Job drawing, mm, ordinate dimensions from the low corner. One solid piece. A direction names the side the tool comes from. Coordinates: 2 decimals unless noted, no trailing zeros. Order: outer loops, then holes, each group sorted by start corner. A loop starts at its lowest first (then second) coordinate and runs counter-clockwise, first axis right, second up. Notation, with made-up numbers: (45.25, 44) - (95.25, 44) arc R27 cw to (95.25, 77) - close; hole circle Ø11 at (-10.75, 73.5). An arc over 180 degrees is marked (long way). Return JSON: item names as keys, results as strings.
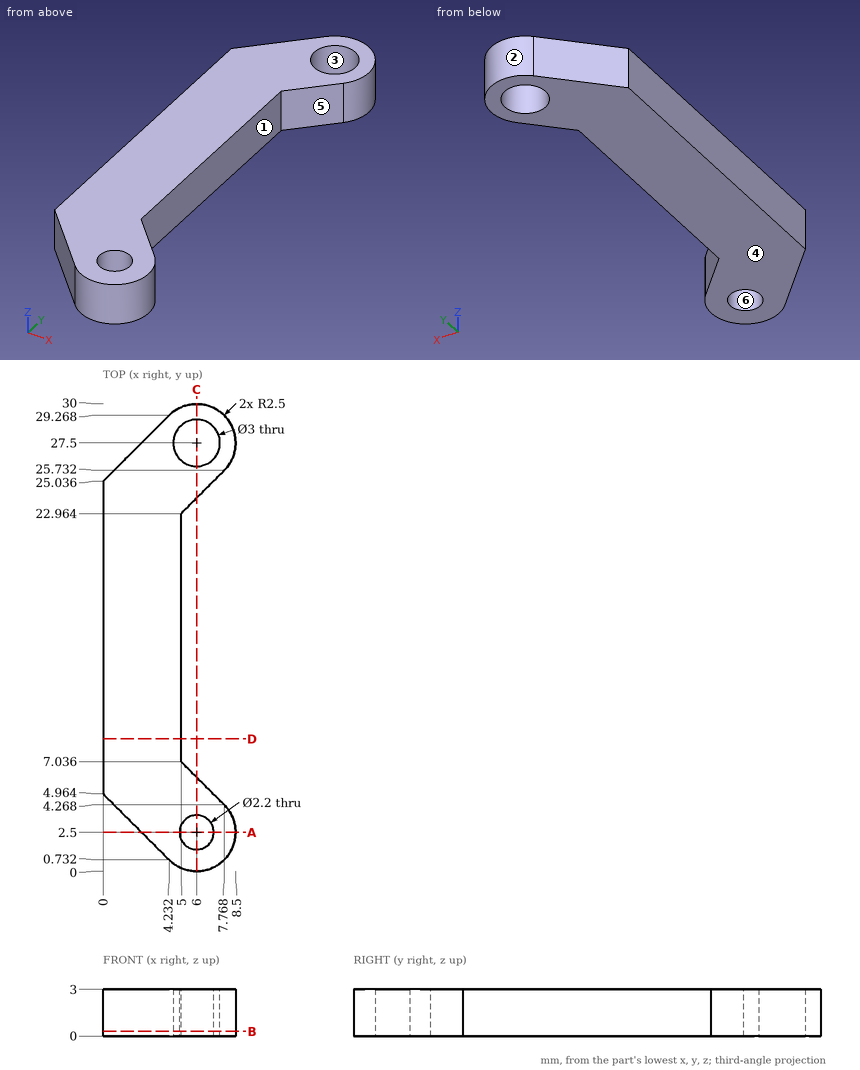
1. Cut at D-D on y = 8.5. Give the cut face in (x, z), plus the area to 3 significant figures.
Check values:
{"outline": "(0, 0) - (5, 0) - (5, 3) - (0, 3) - close", "area": "15.0 mm²"}
2. Mould opens along X. For the marked faces 3, 4, 5 and 6 say: pulls with the +X half, pulls with the -X half, needs draft (parallel to the pull), parting line crosses it, or undercut.
Check values:
{"face 3": "undercut", "face 4": "needs draft", "face 5": "pulls with the +X half", "face 6": "undercut"}
3. Cut at C-C on x = 6. Give the cut face in (y, z) (1 decimal).
Check values:
{"outline": "(0, 0) - (1.4, 0) - (1.4, 3) - (0, 3) - close; (3.6, 0) - (6, 0) - (6, 3) - (3.6, 3) - close; (24, 0) - (26, 0) - (26, 3) - (24, 3) - close; (29, 0) - (30, 0) - (30, 3) - (29, 3) - close"}
4. Drop flat-ended pins along their axis: pin 1 (3.5 mm diameter, centred on x = 6, y = 2.5, fed in from +Z); pin 2 (1 mm diameter, centred on y = 22.5, z = 2.5, fed in from +X) (1 decimal); pin 3 (1.5 mm diameter, centred on y = 24, z = 2, fed in from +X) (1 decimal). Give the stop position or say it passes through.
Check values:
{"pin 1": "z = 3", "pin 2": "x = 5", "pin 3": "x = 6.8"}
5. Cut at B-B on z = 0.3. Give the cut face in (x, y) (1 decimal), plus the area to 3 significant figures.
Check values:
{"outline": "(0, 5) - (4.2, 0.7) arc R2.5 ccw to (7.8, 4.3) - (5, 7) - (5, 23) - (7.8, 25.7) arc R2.5 ccw to (4.2, 29.3) - (0, 25) - close; hole circle Ø3 at (6, 27.5); hole circle Ø2.2 at (6, 2.5)", "area": "148 mm²"}
6. Tool access for the marked faces 1 and 2: list every direction of +Z, -Z, +X, -X, +Y, -Y with a clear straight run to the whole face (end or side of a thin tool).
Check values:
{"face 1": "+Z, -Z, +X", "face 2": "+Z, -Z"}
7. Probe L1, parallel to Y at x = 6, z = 2.1 (1 decimal); L2, parallel to X at y = 25, z = 2.55 (1 decimal); L3, parallel to X at y = 8.5, z = 1.85. List the from-to ranges inside material, lowest first.
Check values:
{"L1": "0 to 1.4, 3.6 to 6, 24 to 26, 29 to 30", "L2": "0 to 7", "L3": "0 to 5"}
8. Cut at A-A on y = 2.5. Give the cut face in (x, z) (1 decimal).
Check values:
{"outline": "(2.5, 0) - (4.9, 0) - (4.9, 3) - (2.5, 3) - close; (7.1, 0) - (8.5, 0) - (8.5, 3) - (7.1, 3) - close"}
